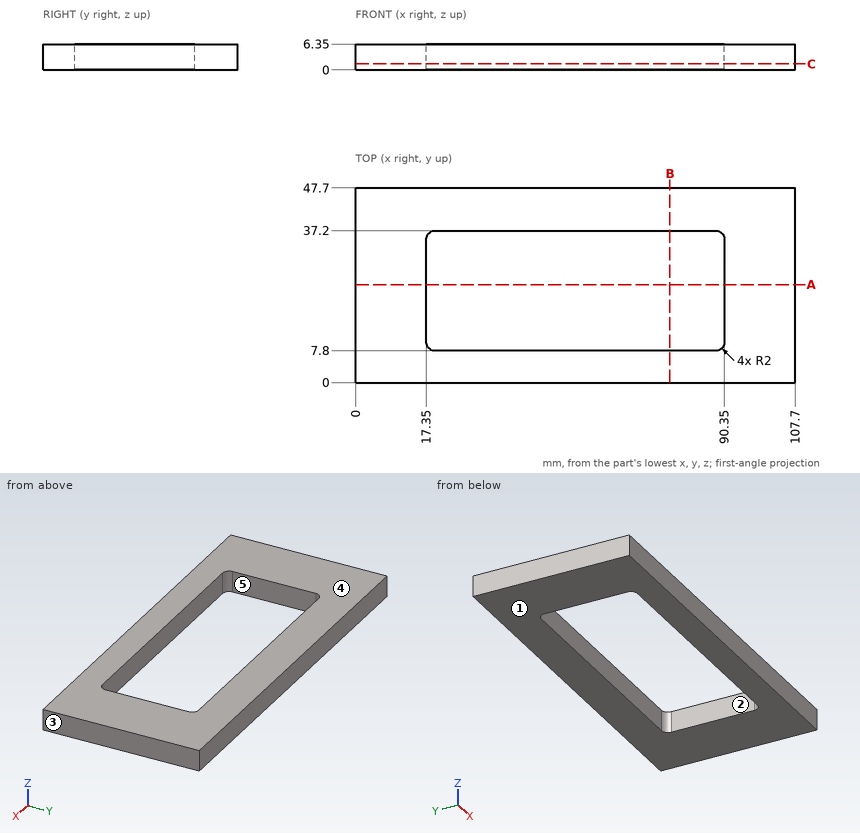
Answer from the drawing. Dimensions are ordinates in mm from the lowest x, y and z of the part. A direction names the side the tool comes from. Round coordinates to 2 decimals unless told otherwise and drop trailing zeros. Loops run counter-clockwise (first coordinate to the right, second up) from the corner with the lowest first, then second, coordinate; pieces in that order, holes last.
Q1. Section C-C on z = 1.5 is taken. Write down the section's boundary in (x, y), and give its area (3 significant figures).
Q2. Section B-B on x = 77 is taken. Write down the section's boundary in (y, z), and give its area (3 significant figures).
Q3. Section A-A on y = 24 is taken. Write down the section's boundary in (x, z).
Q4. This flat-tipped pin is pushed along its axis until it touches: pin 1 (4 mm diameter, centred on x = 30, y = 42.5, fed in from -Z). Where does it stop, or does it pass through?
Q5. Determine the mould class of the marked faces 1, 2 and 3 for opening direction X: released by +X, released by -X, zero draft, split by the parting line, or undercut.
Q6. Consider probe 1 along Y at (x, z) = (73.5, 4.75); probe 2 along X at (y, z) = (26.5, 4.5); probe 3 along X at (y, z) = (36.5, 5). Determine where each line is inside the solid, lowest interval first.
Q7. Which of the six approach directions +Z, -Z, +X, -X, +Y, -Y give full straight-line access (tool end or side, diameter ignored) to the marked faces 4 and 5?
Output:
1. outline: (0, 0) - (107.7, 0) - (107.7, 47.7) - (0, 47.7) - close; hole (17.35, 9.8) arc R2 ccw to (19.35, 7.8) - (88.35, 7.8) arc R2 ccw to (90.35, 9.8) - (90.35, 35.2) arc R2 ccw to (88.35, 37.2) - (19.35, 37.2) arc R2 ccw to (17.35, 35.2) - close
1. area: 2,990 mm2
2. outline: (0, 0) - (7.8, 0) - (7.8, 6.35) - (0, 6.35) - close; (37.2, 0) - (47.7, 0) - (47.7, 6.35) - (37.2, 6.35) - close
2. area: 116 mm2
3. outline: (0, 0) - (17.35, 0) - (17.35, 6.35) - (0, 6.35) - close; (90.35, 0) - (107.7, 0) - (107.7, 6.35) - (90.35, 6.35) - close
4. pin 1: stops at z = 0
5. face 1: zero draft
5. face 2: undercut
5. face 3: released by +X
6. probe 1: y = 0 to 7.8, 37.2 to 47.7
6. probe 2: x = 0 to 17.35, 90.35 to 107.7
6. probe 3: x = 0 to 17.83, 89.87 to 107.7
7. face 4: +Z, +X, -X, +Y, -Y
7. face 5: +Z, -Z
